Input: part model. Units: mm. Frame: model coordinates. A direction names the side the tool comes from. Round coordinates to 2 decimals unless told otherwise and drop trailing zeros. Loops run counter-clockwise (first coordinate to the right, second up) from the corner with the lowest first, then second, coordinate; pieces in that order, holes last.
(1) First-contact query: pin 1 Ø3 at (y, z) = (-3.5, 18) entering from -X; pin 2 Ø2 at (y, z) = (-2, 13) entering from +X; pin 3 Ø3 at (x, y) = (0, 0) entering from -Z; pin 4 Ø2 at (y, z) = (1, 17.5) entering from -X. Flat tips, straight axial feed; report the tip coordinate or a pass-through.
(2) Cut plane D-D, the plane z = 2. Output: boundary loops of the cut face in (x, y), and give its area (3 significant figures).
(3) Access query for faces 1 (the face through (-1.216, -1.115, 3.698)), 2 (the face through (0, 0, 21)). Directions: +Z, -Z, +X, -X, +Y, -Y. A direction counts if a zero-diameter tool reaches every point of the face in a straight line with its end or side. Return the directions, or none.
(4) Draft query along Y for faces 3 (the face through (2, 0, 0)), 4 (the face through (-3.54, 3.24, 10.35)), 5 (the face through (0, 0, 7.5)). Return one class per face: released by +Y, released by -Y, zero draft, split by the parting line, or undercut.
(5) Cut plane C-C, the plane z = 8.75. Output: boundary loops of the cut face in (x, y).
(6) Line query: line 1 (Y direction, x = 0, z = 2.25); line 2 (Z direction, x = -0.75, y = -4.25); line 3 (Y direction, x = -2.75, z = 18.5). Output: solid intervals per line, ascending.
(7) Cut plane A-A, the plane x = 0. Output: boundary loops of the cut face in (y, z).
(8) Cut plane B-B, the plane y = -1. Output: boundary loops of the cut face in (x, z), and give its area (3 significant figures).
from build123d import *

# Parameters (mm, degrees)
F0_R          = 4.8
F1_DEPTH      = 21
F2_R          = 1.65
F3_DEPTH      = 7.5
F5_DEPTH      = 4.8010001002
F5_DEPTH_BACK = 4.8010001002


with BuildPart() as f1:
    # F0 (on Top) → F1 (new body)
    with BuildSketch(Plane.XY):
        Circle(F0_R)
    extrude(amount=F1_DEPTH)

    # F2 (on face) → F3 (cut)
    with BuildSketch(Plane(origin=(0, 0, 0), x_dir=(1, 0, 0), z_dir=(0, 0, -1))):
        Circle(F2_R)
    extrude(amount=-F3_DEPTH, mode=Mode.SUBTRACT)

    # F4 (on Front) → F5 (cut, two sides)
    with BuildSketch(Plane.XZ) as f5_sk:
        with BuildLine():
            Line((2.7497246979, 15.8889112544), (2.7497298501, 15.8114545531))
            ThreePointArc((2.7497298501, 15.8114545531), (2.7499999939, 15.8501829219), (2.7497246979, 15.8889112544))
        make_face()
        with BuildLine():
            Line((2.7499999939, 11.7501829219), (2.7497298501, 15.8114545531))
            Line((2.7497298501, 15.8114545531), (2.7497246979, 15.8889112544))
            ThreePointArc((2.7497246979, 15.8889112544), (-0.0195165469, 18.5999307454), (-2.7499999973, 15.8498791315))
            Line((-2.7499999973, 15.8498791315), (-2.7498211771, 11.781360704))
            Line((-2.7498211771, 11.781360704), (-2.7498184098, 11.718397575))
            ThreePointArc((-2.7498184098, 11.718397575), (0.0158929328, 9.000045925), (2.7499999939, 11.7501829219))
        make_face()
        with BuildLine():
            ThreePointArc((-2.7498211771, 11.781360704), (-2.7499999973, 11.7498791315), (-2.7498184098, 11.718397575))
            Line((-2.7498184098, 11.718397575), (-2.7498211771, 11.781360704))
        make_face()
    extrude(amount=-F5_DEPTH, mode=Mode.SUBTRACT)
    extrude(f5_sk.sketch, amount=F5_DEPTH_BACK, mode=Mode.SUBTRACT)


solid = f1.part
Reported:
1. pin 1: stops at x = -4.36
1. pin 2: stops at x = 4.69
1. pin 3: stops at z = 7.5
1. pin 4: stops at x = -4.8
2. outline: circle Ø9.6 at (0, 0); hole circle Ø3.3 at (0, 0)
2. area: 63.8 mm2
3. face 1: -Z
3. face 2: +Z, +X, -X, +Y, -Y
4. face 3: zero draft
4. face 4: split by the parting line
4. face 5: undercut
5. outline: circle Ø9.6 at (0, 0)
6. line 1: y = -4.8 to -1.65, 1.65 to 4.8
6. line 2: z = 0 to 9.1, 18.5 to 21
6. line 3: y = -3.93 to 3.93
7. outline: (-4.8, 0) - (-1.65, 0) - (-1.65, 7.5) - (1.65, 7.5) - (1.65, 0) - (4.8, 0) - (4.8, 9) - (-4.8, 9) - close; (-4.8, 18.6) - (4.8, 18.6) - (4.8, 21) - (-4.8, 21) - close
8. outline: (-4.69, 0) - (-1.31, 0) - (-1.31, 7.5) - (1.31, 7.5) - (1.31, 0) - (4.69, 0) - (4.69, 21) - (-4.69, 21) - close; hole (-2.75, 11.78) arc R2.75 ccw (long way) to (2.75, 11.75) - (2.75, 15.81) arc R2.75 ccw (long way) to (-2.75, 15.85) - close
8. area: 131 mm2
